```python
from build123d import *

# Parameters (mm, degrees)
SALIENTE_EXTRUIR1_OUTLINE_R = 2.1
SALIENTE_EXTRUIR1_DEPTH     = 50
REDONDEO1_R                 = 1.5
REDONDEO2_R                 = 0.2
CROQUIS2_R                  = 2.5
CORTAR_EXTRUIR1_DEPTH       = 55.772255751


# Read off the part's stored shape, not the designer's step: Saliente-Extruir1
with BuildPart() as part:
    # Saliente-Extruir1 outline → Saliente-Extruir1 (new body)
    with BuildSketch(Plane(origin=(0, 0, 0), x_dir=(1, 0, 0), z_dir=(0, 1, 0))):
        Polygon((-5.539339828, -6.6), (-2.84, -3.900660172), (2.84, -3.900660172), (5.539339828, -6.6), (5.539339828, -8.2), (3.1, -8.2), (4.9, -10), (10, -10), (10, -4.9), (8.2, -3.1), (8.2, -5.539339828), (6.6, -5.539339828), (3.900660172, -2.84), (3.900660172, 2.84), (6.6, 5.539339828), (8.2, 5.539339828), (8.2, 3.1), (10, 4.9), (10, 10), (4.9, 10), (3.1, 8.2), (5.539339828, 8.2), (5.539339828, 6.6), (2.84, 3.900660172), (-2.84, 3.900660172), (-5.539339828, 6.6), (-5.539339828, 8.2), (-3.1, 8.2), (-4.9, 10), (-10, 10), (-10, 4.9), (-8.2, 3.1), (-8.2, 5.539339828), (-6.6, 5.539339828), (-3.900660172, 2.84), (-3.900660172, -2.84), (-6.6, -5.539339828), (-8.2, -5.539339828), (-8.2, -3.1), (-10, -4.9), (-10, -10), (-4.9, -10), (-3.1, -8.2), (-5.539339828, -8.2), align=None)
        Circle(SALIENTE_EXTRUIR1_OUTLINE_R, mode=Mode.SUBTRACT)
    extrude(amount=SALIENTE_EXTRUIR1_DEPTH)

    # Redondeo1
    redondeo1_edges = [part.edges().sort_by_distance(p)[0] for p in [
        (-10, 25, 10),
        (-10, 25, -10),
        (10, 25, -10),
        (10, 25, 10),
    ]]
    fillet(redondeo1_edges, radius=REDONDEO1_R)

    # Redondeo2
    redondeo2_edges = [part.edges().sort_by_distance(p)[0] for p in [
        (-5.539339828, 25, 8.2),
        (-3.1, 25, 8.2),
        (-8.2, 25, 3.1),
        (-8.2, 25, 5.539339828),
        (-8.2, 25, -5.539339828),
        (-8.2, 25, -3.1),
        (-3.1, 25, -8.2),
        (-5.539339828, 25, -8.2),
        (5.539339828, 25, -8.2),
        (3.1, 25, -8.2),
        (8.2, 25, -3.1),
        (8.2, 25, -5.539339828),
        (8.2, 25, 5.539339828),
        (8.2, 25, 3.1),
        (3.1, 25, 8.2),
        (5.539339828, 25, 8.2),
    ]]
    fillet(redondeo2_edges, radius=REDONDEO2_R)

    # Croquis2 → Cortar-Extruir1 (cut, through all)
    with BuildSketch(Plane(origin=(0, 0, -10), x_dir=(-1, 0, 0), z_dir=(0, 0, -1))):
        with Locations((0, 40)):
            Circle(CROQUIS2_R)
        with Locations((0, 10)):
            Circle(CROQUIS2_R)
    extrude(amount=-CORTAR_EXTRUIR1_DEPTH, mode=Mode.SUBTRACT)


solid = part.part
```
Geometry: final body of the model. Coordinates: model frame, mm. A direction names the side the tool comes from. Coordinates: 2 decimals unless noted, no trailing zeros. Write each loop counter-clockwise with the first axis right and the second up, starting at its lowest first coordinate (ties: lowest second). Pieces come first, ordered by that corner, then holes. Notation, with made-up numbers: M 30,-35 L 43,-35 A26 cw 43,-4 Z; hole C 22,32.5 d11. An arc over 180 degrees is marked long. Use CSV: the item, a comma, the result in double quotes. Start each with the question number.
1. First-contact query: P1, Ø1.5, axis at y = 15, z = -0.5, coming from the -X side; P2, Ø0.9, axis at y = 29, z = 4, coming from the +X side; P3, Ø0.5, axis at y = 15.5, z = -4.5, coming from the -X side; P4, Ø1.9, axis at y = 35.5, z = 4, coming from the -X side. Flat tips, straight axial feed; report the tip coordinate or a pass-through.
2. Mould query, pull axis Z, two halves, no side actions, for faces 4 (the face through (4.21, 24.65, -5.27)), 5 (the face through (8.2, 25, 4)), 6 (the face through (-7, 25, 10)), 7 (the face through (-9.57, 25.35, -9.55)). Classes: pulls with the +Z half, pulls with the -Z half, needs draft (parallel to the pull), parting line crosses it, or undercut.
3. Cut plane A-A on x = 0. Return the cut outline in (y, z), plus the area to 3 significant figures.
4. Reachability of faces 1 (the face through (9.3, 24.6, -4.2)), 2 (the face through (0, 25, 3.901)), 3 (the face through (-4.21, 24.65, 5.27)) from +Z, -Z, +X, -X, +Y, -Y: full face, straight path, thin tool, end or side. Return the list, or none.
5. Ray query, probe 1 along X at (y, z) = (37, -7.25); probe 2 along Z at (x, y) = (3.5, 3.5); probe 3 along X at (y, z) = (14, -4). Return the intervals inside material, ascending.
6. Cut plane B-B on z = 0. Return the cut outline in (x, y), plus the area to 3 significant figures.
Entries:
1,P1,"x = -3.9"
1,P2,"x = 9.55"
1,P3,"x = -9.85"
1,P4,"x = -10"
2,face 4,"undercut"
2,face 5,"undercut"
2,face 6,"pulls with the +Z half"
2,face 7,"pulls with the -Z half"
3,outline,"M 0,-3.9 L 7.5,-3.9 L 7.5,-2.1 L 0,-2.1 Z; M 0,2.1 L 7.5,2.1 L 7.5,3.9 L 0,3.9 Z; M 12.5,-3.9 L 37.5,-3.9 L 37.5,-2.1 L 12.5,-2.1 Z; M 12.5,2.1 L 37.5,2.1 L 37.5,3.9 L 12.5,3.9 Z; M 42.5,-3.9 L 50,-3.9 L 50,-2.1 L 42.5,-2.1 Z; M 42.5,2.1 L 50,2.1 L 50,3.9 L 42.5,3.9 Z"
3,area,"144 mm²"
4,face 1,"+X, +Y, -Y"
4,face 2,"+Z, +Y, -Y"
4,face 3,"+Y, -Y"
5,probe 1,"-10 to -5.54, 5.54 to 10"
5,probe 2,"-8.6 to -8.22, -4.56 to 4.56, 8.22 to 8.6"
5,probe 3,"-9.1 to -8.2, -5.06 to -2.94, 2.94 to 5.06, 8.2 to 9.1"
6,outline,"M -3.9,0 L -2.1,0 L -2.1,8.64 A2.5 cw -2.1,11.36 L -2.1,38.64 A2.5 cw -2.1,41.36 L -2.1,50 L -3.9,50 Z; M 2.1,0 L 3.9,0 L 3.9,50 L 2.1,50 L 2.1,41.36 A2.5 cw 2.1,38.64 L 2.1,11.36 A2.5 cw 2.1,8.64 Z"
6,area,"177 mm²"
